Verification items for the finished model (mm, model axes). A direction names the side the tool comes from. Round coordinates to 2 decimals unless told otherwise and drop trailing zeros. Loops run counter-clockwise (first coordinate to the right, second up) from the corner with the lowest first, then second, coordinate; pieces in that order, holes last. Notation, with made-up numbers: M 75.25,47 L 111.25,47 A21 ccw 111.25,72 Z; hole C 74,23.25 d9. An arc over 180 degrees is marked long. Answer as CSV lines item,"result".
```python
from build123d import *

# Parameters (mm, degrees)
SKETCH1_R                   = 57.15
BOSS_EXTRUDE1_DEPTH         = 19.05
F_1_4_CLEARANCE_HOLE1_D     = 6.7564
F_1_4_CLEARANCE_HOLE1_DEPTH = 57.15
F_1_4_CLEARANCE_HOLE1_TIP   = 2.029827343
SKETCH9_R                   = 44.45
PIPE_ALIGNMENTSEAL_DEPTH    = 2.38125


with BuildPart() as part:
    # Sketch1 → Boss-Extrude1 (new body)
    with BuildSketch(Plane.XY):
        with Locations(Location((0, 0, 0), (0, 0, 180))):
            Circle(SKETCH1_R)
    extrude(amount=BOSS_EXTRUDE1_DEPTH)

    # 1/4 Clearance Hole1
    with Locations(Plane.XY.offset(19.05)):
        with Locations((0, 50.8), (29.859490816, 41.098063314), (48.313671028, 15.698063314), (48.313671028, -15.698063314), (29.859490816, -41.098063314), (0, -50.8), (-29.859490816, -41.098063314), (-48.313671028, -15.698063314), (-48.313671028, 15.698063314), (-29.859490816, 41.098063314)):
            Hole(F_1_4_CLEARANCE_HOLE1_D / 2, depth=F_1_4_CLEARANCE_HOLE1_DEPTH)
            with Locations((0, 0, -(F_1_4_CLEARANCE_HOLE1_DEPTH + F_1_4_CLEARANCE_HOLE1_TIP / 2))):  # 118° drill point
                Cone(0, F_1_4_CLEARANCE_HOLE1_D / 2, F_1_4_CLEARANCE_HOLE1_TIP, mode=Mode.SUBTRACT)

    # Sketch9 → Pipe AlignmentSeal (add)
    with BuildSketch(Plane(origin=(0, 0, 0), x_dir=(-1, 0, 0), z_dir=(0, 0, -1))):
        with Locations(Location((0, 0, 0), (0, 0, 180))):
            Circle(SKETCH9_R)
    extrude(amount=PIPE_ALIGNMENTSEAL_DEPTH)

    # Sketch14 → 1/2 NPT Tapped Hole6 (revolve, cut)
    with BuildSketch(Plane(origin=(0, 0, 19.05), x_dir=(0, -1, 0), z_dir=(1, 0, 0))):
        Polygon((0, 0), (0, 21.43125), (9.5631, 21.43125), (8.9281, 20.79625), (8.9281, 19.05), (10.275764385, 19.05), (10.8320459, 0.4709541), (11.303, 0), align=None)
    revolve(axis=Axis((0, 0, 25.4), (0, 0, -1)), mode=Mode.SUBTRACT)


solid = part.part
```
1) Section check B-B (y = 0). Record the cut outline in (x, z).
Here are the results:
outline,"M -57.15,0 L -44.45,0 L -44.45,-2.38 L -9.56,-2.38 L -8.93,-1.75 L -8.93,0 L -10.28,0 L -10.83,18.58 L -11.3,19.05 L -57.15,19.05 Z; M 8.93,-1.75 L 9.56,-2.38 L 44.45,-2.38 L 44.45,0 L 57.15,0 L 57.15,19.05 L 11.3,19.05 L 10.83,18.58 L 10.28,0 L 8.93,0 Z"
2) Set-up check for faces 1 (the cylindrical face through (-32.8, -30, -1.2)), 2 (the cylindrical face through (49.05, 12.4, 9.39)), 3 (the flat face through (-5, -8, 0)): record each of +Z, -Z, +X, -X, +Y, -Y from which the full face is reachable in a straight line by a thin tool's end or side.
Here are the results:
face 1,"-Z"
face 2,"+Z, -Z"
face 3,"+Z"
3) Section check C-C (z = 8). State how many separate pieces and enclosed holes the cut face has, plus the area to 3 significant figures.
Here are the results:
separate pieces,"1"
enclosed holes,"11"
area,"9,550 mm^2"
4) Section check A-A (x = 0). Record the cut outline in (y, z).
Here are the results:
outline,"M -57.15,0 L -54.18,0 L -54.18,19.05 L -57.15,19.05 Z; M -47.42,0 L -44.45,0 L -44.45,-2.38 L -9.56,-2.38 L -8.93,-1.75 L -8.93,0 L -10.28,0 L -10.83,18.58 L -11.3,19.05 L -47.42,19.05 Z; M 8.93,-1.75 L 9.56,-2.38 L 44.45,-2.38 L 44.45,0 L 47.42,0 L 47.42,19.05 L 11.3,19.05 L 10.83,18.58 L 10.28,0 L 8.93,0 Z; M 54.18,0 L 57.15,0 L 57.15,19.05 L 54.18,19.05 Z"
5) Go/stop test with flat-tipped pins: pin 1 (11 mm diameter, centred on x = 48.31, y = -15.7, fed in from -Z); pin 2 (23 mm diameter, centred on x = 0, y = 0, fed in from -Z); pin 3 (4 mm diameter, centred on y = -42, z = 12, fed in from -X); pin 4 (1.5 mm diameter, centred on x = 38.5, z = 14.5, fed in from -Y). Record where each tip stops, or that it passes through.
Here are the results:
pin 1,"stops at z = 0"
pin 2,"stops at z = -2.38"
pin 3,"stops at x = -40.82"
pin 4,"stops at y = -42.91"
6) Material ranges on probe 1 along X at (y, z) = (-38.5, 2); probe 2 along Y at (x, z) = (0, -0.35); probe 3 along Y at (x, z) = (-32, 8.75), recorded low to high.
Here are the results:
probe 1,"x = -42.24 to -32.02, -27.7 to 27.7, 32.02 to 42.24"
probe 2,"y = -44.45 to -8.93, 8.93 to 44.45"
probe 3,"y = -47.35 to -43.71, -38.48 to 38.48, 43.71 to 47.35"
7) Section check D-D (y = -50.8). Record the cut outline in (x, z).
Here are the results:
outline,"M -26.18,0 L -3.38,0 L -3.38,19.05 L -26.18,19.05 Z; M 3.38,0 L 26.18,0 L 26.18,19.05 L 3.38,19.05 Z"
